Answer from the drawing. Dimensions are ordinates in mm from the lowest x, y and z of the part. A direction names the side the tool comes from. Coordinates: 2 decimals unless noted, no trailing zeros. Write each loop counter-clockwise with the first axis right and the second up, starting at its lowest first coordinate (ties: lowest second). Pieces come first, ordered by that corner, then holes. Notation, with made-up numbers: (66, 8.25) -> (124, 8.25) arc R30 ccw to (124, 36.25) -> close; hole circle Ø6 at (88, 80.5). An arc over 180 degrees is marked (long way). Answer as a JSON object with one key per item and string values. Group by question number.
(1) Find section A-A (y = 12.5). Give the vertices of the cut face in (x, z).
(2) Flat-ended cylindrical pins translate along their axes: P1, Ø1.7, axis at y = 13.5, z = 2.5, coming from the -X side; P2, Ø2.5, axis at y = 12.5, z = 4.2, coming from the -X side. Find the tip coordinate at first contact, or state that the pin passes through.
(3) Which of the six approach directions +Z, -Z, +X, -X, +Y, -Y give full straight-line access (tool end or side, diameter ignored) to the marked faces 4 and 5?
(4) Find section D-D (y = 8.75). Give the vertices of the cut face in (x, z), then the cut area to 3 significant figures.
(5) Find section B-B (x = 9). Give the vertices of the cut face in (y, z), then the cut area to 3 significant figures.
(6) Find section C-C (z = 8). Give the vertices of the cut face in (x, y).
(7) For a pull along X with two mould halves and no side action, classify the marked faces 1, 2 and 3 as +X half, -X half, draft (parallel to the pull), parting line (faces both ways), or undercut.
(8) Straight lines are drawn through the part: L1, parallel to Y at x = 12.5, z = 5.25; L2, parallel to Z at x = 1.8, y = 12.5; L3, parallel to X at y = 10, z = 3.75. For each, find the intervals that lie inside material, in ascending order.
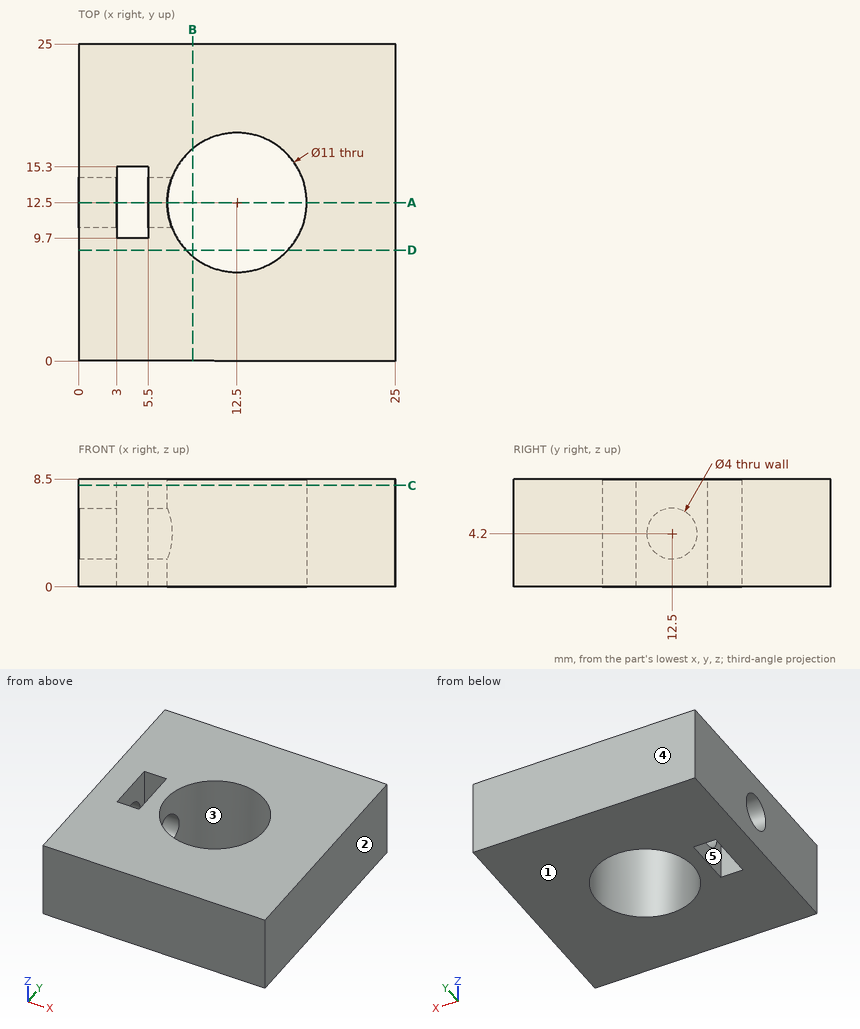
Results below:
{
 "1": {"outline": "(0, 0) -> (3, 0) -> (3, 2.2) -> (0, 2.2) -> close; (0, 6.2) -> (3, 6.2) -> (3, 8.5) -> (0, 8.5) -> close; (5.5, 0) -> (7, 0) -> (7, 2.2) -> (5.5, 2.2) -> close; (5.5, 6.2) -> (7, 6.2) -> (7, 8.5) -> (5.5, 8.5) -> close; (18, 0) -> (25, 0) -> (25, 8.5) -> (18, 8.5) -> close"},
 "2": {"P1": "stops at x = 0", "P2": "stops at x = 17.86"},
 "3": {"face 4": "+Z, -Z, +X, -X, +Y", "face 5": "+Z, -Z"},
 "4": {"outline": "(0, 0) -> (8.48, 0) -> (8.48, 8.5) -> (0, 8.5) -> close; (16.52, 0) -> (25, 0) -> (25, 8.5) -> (16.52, 8.5) -> close", "area": "144 mm2"},
 "5": {"outline": "(0, 0) -> (8.26, 0) -> (8.26, 8.5) -> (0, 8.5) -> close; (16.74, 0) -> (25, 0) -> (25, 8.5) -> (16.74, 8.5) -> close", "area": "140 mm2"},
 "6": {"outline": "(0, 0) -> (25, 0) -> (25, 25) -> (0, 25) -> close; hole (3, 9.7) -> (5.5, 9.7) -> (5.5, 15.3) -> (3, 15.3) -> close; hole circle Ø11 at (12.5, 12.5)"},
 "7": {"face 1": "draft", "face 2": "+X half", "face 3": "undercut"},
 "8": {"L1": "y = 0 to 7, 18 to 25", "L2": "z = 0 to 2.2, 6.2 to 8.5", "L3": "x = 0 to 3, 5.5 to 7.6, 17.4 to 25"}
}
